Part model, mm, in its own coordinate system. Coordinates: 2 decimals unless noted, no trailing zeros. Loops run counter-clockwise (first coordinate to the right, second up) from the corner with the lowest first, then second, coordinate; pieces in that order, holes last. Notation, with made-up numbers: M 60.5,52.5 L 103.5,52.5 A32 cw 103.5,83.5 Z; hole C -10,11.25 d3. An arc over 180 degrees is marked long. Use a Markdown table: item, result. Add a question column.
1) Pull direction X, two halves, no side cores. Call faces 1 (the flat face through (-1, -15, -47)), 2 (the cylindrical face through (83.624, -14.79, -40.996)): released by +X, released by -X, zero draft, split by the parting line, or undercut.
2) Band-saw the part on C-C (z = 37). State how many separate pieces and enclosed holes the cut face has, plus the area to 3 significant figures.
3) Wall check: probe 1 along X at (y, z) = (-22, 37); probe 2 along Z at (x, y) = (83.8, -11.75); probe 3 along Z at (x, y) = (83, -22). Give the ranges that are in metal, low to high. Write a range as from..to.
4) Band-saw the part on B-B (x = -26). List the corners of the cut face in (y, z), plus the area to 3 significant figures.
5) Band-saw the part on A-A (x = -83.8). List the corners of the cut face in (y, z) (3 decimals).
6) Pin check, flat tip, straight feed: pin 1 Ø8 at (x, z) = (0, 37) entering from +Y (3 decimals). Stop position of the tip, or through.
from build123d import *

# Parameters (mm, degrees)
SKETCH1_W                      = 221.6
SKETCH1_H                      = 94
BOSS_EXTRUDE1_DEPTH            = 30
SKETCH2_R                      = 5.12
CUT_EXTRUDE1_DEPTH             = 125.038864877
CHAMFER1_SIZE                  = 1
M5_TAPPED_HOLE1_D              = 4.2
M5_TAPPED_HOLE1_DEPTH          = 14
M5_TAPPED_HOLE1_TIP            = 1.2618073
M8_TAPPED_HOLE1_AT_2_COUNT     = 2
M8_TAPPED_HOLE1_AT_2_PITCH     = 74
M8_TAPPED_HOLE1_AT_3_COUNT     = 2
M8_TAPPED_HOLE1_AT_3_PITCH     = 214.752322455
M8_TAPPED_HOLE1_AT_4_COUNT     = 2
M8_TAPPED_HOLE1_AT_4_PITCH     = 201.6
M8_TAPPED_HOLE1_AT_5_COUNT     = 2
M8_TAPPED_HOLE1_AT_5_PITCH     = 100.8
M8_TAPPED_HOLE1_AT_6_COUNT     = 2
M8_TAPPED_HOLE1_AT_6_PITCH     = 125.046551332
F_8_0MM_DOWEL_HOLE1_AT_2_COUNT = 2
F_8_0MM_DOWEL_HOLE1_AT_2_PITCH = 183.209606735


with BuildPart() as part:
    # Sketch1 → Boss-Extrude1 (new body)
    with BuildSketch(Plane(origin=(0, 0, 0), x_dir=(1, 0, 0), z_dir=(0, 1, 0))):
        Rectangle(SKETCH1_W, SKETCH1_H)
    extrude(amount=-BOSS_EXTRUDE1_DEPTH)

    # Sketch2 → Cut-Extrude1 (cut, through all)
    with BuildSketch(Plane(origin=(0, 0, 0), x_dir=(1, 0, 0), z_dir=(0, 1, 0))):
        with Locations(Location((35.8, 0, 0), (0, 0, 270))):
            Circle(SKETCH2_R)
        with Locations(Location((73.8, 0, 0), (0, 0, 270))):
            Circle(SKETCH2_R)
        with BuildLine():
            Line((-33.8, 15), (4.2, 15))
            ThreePointArc((4.2, 15), (19.2, 0), (4.2, -15))
            Line((4.2, -15), (-33.8, -15))
            ThreePointArc((-33.8, -15), (-48.8, 0), (-33.8, 15))
        make_face()
    extrude(amount=-CUT_EXTRUDE1_DEPTH, mode=Mode.SUBTRACT)

    # Cut-Sweep1: sweep along a curve in space
    with BuildLine() as cut_sweep1_path:
        ThreePointArc((-33.8, 0, 15), (-48.8, 0, 0), (-33.8, 0, -15))
        Line((-33.8, 0, -15), (4.2, 0, -15))
        ThreePointArc((4.2, 0, -15), (19.2, 0, 0), (4.2, 0, 15))
        Line((4.2, 0, 15), (-33.8, 0, 15))
    # Sketch3 → Cut-Sweep1 (sweep, cut)
    with BuildSketch(Plane(origin=(-14.8, 0, 0), x_dir=(0, 0, -1), z_dir=(1, 0, 0))):
        Polygon((15, -3), (15.707019882, -30), (15, -30), align=None)
    sweep(path=cut_sweep1_path.line, mode=Mode.SUBTRACT)

    # Cut-Sweep2: sweep along a curve in space
    with BuildLine() as cut_sweep2_path:
        ThreePointArc((35.8, 0, 5.12), (39.42038672, 0, 3.62038672), (40.92, 0, 0))
        ThreePointArc((40.92, 0, 0), (39.42038672, 0, -3.62038672), (35.8, 0, -5.12))
        ThreePointArc((35.8, 0, -5.12), (32.17961328, 0, -3.62038672), (30.68, 0, 0))
        ThreePointArc((30.68, 0, 0), (32.17961328, 0, 3.62038672), (35.8, 0, 5.12))
    # Sketch5 → Cut-Sweep2 (sweep, cut)
    with BuildSketch(Plane.XY):
        Polygon((40.92, -3), (41.627019882, -30), (40.92, -30), align=None)
    sweep(path=cut_sweep2_path.line, mode=Mode.SUBTRACT)

    # Cut-Sweep3: sweep along a curve in space
    with BuildLine() as cut_sweep3_path:
        ThreePointArc((73.8, 0, 5.12), (77.42038672, 0, 3.62038672), (78.92, 0, 0))
        ThreePointArc((78.92, 0, 0), (77.42038672, 0, -3.62038672), (73.8, 0, -5.12))
        ThreePointArc((73.8, 0, -5.12), (70.17961328, 0, -3.62038672), (68.68, 0, 0))
        ThreePointArc((68.68, 0, 0), (70.17961328, 0, 3.62038672), (73.8, 0, 5.12))
    # Sketch9 → Cut-Sweep3 (sweep, cut)
    with BuildSketch(Plane.XY):
        Polygon((78.92, -3), (79.627019882, -30), (78.92, -30), align=None)
    sweep(path=cut_sweep3_path.line, mode=Mode.SUBTRACT)

    # Chamfer1
    chamfer1_edges = [part.edges().sort_by_distance(p)[0] for p in [
        (-110.8, -30, 0),
        (0, -30, 47),
        (110.8, -30, 0),
        (0, 0, 47),
        (-110.8, 0, 0),
        (0, 0, -47),
        (110.8, 0, 0),
        (110.8, -15, 47),
        (-110.8, -15, 47),
        (-110.8, -15, -47),
        (0, -30, -47),
    ]]
    chamfer(chamfer1_edges, length=CHAMFER1_SIZE)

    # M5 Tapped Hole1
    with Locations(Plane.XY.offset(47)):
        with Locations((14.45, -7)):
            Hole(M5_TAPPED_HOLE1_D / 2, depth=M5_TAPPED_HOLE1_DEPTH)
            with Locations((0, 0, -(M5_TAPPED_HOLE1_DEPTH + M5_TAPPED_HOLE1_TIP / 2))):  # 118° drill point
                Cone(0, M5_TAPPED_HOLE1_D / 2, M5_TAPPED_HOLE1_TIP, mode=Mode.SUBTRACT)

    # Sketch15 → M8 Tapped Hole1 (revolve, cut)
    with BuildSketch(Plane(origin=(-100.8, 0, 37), x_dir=(0, 0, 1), z_dir=(1, 0, 0))):
        Polygon((0, 0), (0, 30), (4.025, 30), (3.4, 29.375), (3.4, 0.625), (4.025, 0), align=None)
    m8_tapped_hole1 = revolve(axis=Axis((-100.8, 6.35, 37), (0, -1, 0)), mode=Mode.SUBTRACT)

    # M8 Tapped Hole1 at 2: M8 Tapped Hole1 ×2
    with Locations(*[(0, 0, -i * M8_TAPPED_HOLE1_AT_2_PITCH) for i in range(1, M8_TAPPED_HOLE1_AT_2_COUNT)]):
        add(m8_tapped_hole1, mode=Mode.SUBTRACT)

    # M8 Tapped Hole1 at 3: M8 Tapped Hole1 ×2
    with Locations(*[Vector(0.9387558546280332, 0, -0.34458300219481375) * (i * M8_TAPPED_HOLE1_AT_3_PITCH) for i in range(1, M8_TAPPED_HOLE1_AT_3_COUNT)]):
        add(m8_tapped_hole1, mode=Mode.SUBTRACT)

    # M8 Tapped Hole1 at 4: M8 Tapped Hole1 ×2
    with Locations(*[(i * M8_TAPPED_HOLE1_AT_4_PITCH, 0, 0) for i in range(1, M8_TAPPED_HOLE1_AT_4_COUNT)]):
        add(m8_tapped_hole1, mode=Mode.SUBTRACT)

    # M8 Tapped Hole1 at 5: M8 Tapped Hole1 ×2
    with Locations(*[(i * M8_TAPPED_HOLE1_AT_5_PITCH, 0, 0) for i in range(1, M8_TAPPED_HOLE1_AT_5_COUNT)]):
        add(m8_tapped_hole1, mode=Mode.SUBTRACT)

    # M8 Tapped Hole1 at 6: M8 Tapped Hole1 ×2
    with Locations(*[Vector(0.8060997998454218, 0, -0.591779614965885) * (i * M8_TAPPED_HOLE1_AT_6_PITCH) for i in range(1, M8_TAPPED_HOLE1_AT_6_COUNT)]):
        add(m8_tapped_hole1, mode=Mode.SUBTRACT)

    # Sketch17 → Ø8.0mm Dowel Hole1 (revolve, cut)
    with BuildSketch(Plane(origin=(-83.8, 0, 37), x_dir=(0, 0, 1), z_dir=(1, 0, 0))):
        Polygon((0, 0), (0, 30), (4.025, 30), (4, 29.975), (4, 0.025), (4.025, 0), align=None)
    f_8_0mm_dowel_hole1 = revolve(axis=Axis((-83.8, 6.35, 37), (0, -1, 0)), mode=Mode.SUBTRACT)

    # Ø8.0mm Dowel Hole1 at 2: Ø8.0mm Dowel Hole1 ×2
    with Locations(*[Vector(0.9147991908656035, 0, -0.40390895062085114) * (i * F_8_0MM_DOWEL_HOLE1_AT_2_PITCH) for i in range(1, F_8_0MM_DOWEL_HOLE1_AT_2_COUNT)]):
        add(f_8_0mm_dowel_hole1, mode=Mode.SUBTRACT)

    # Mirror1: Ø8.0mm Dowel Hole1 across plane
    add(f_8_0mm_dowel_hole1.mirror(Plane.XY), mode=Mode.SUBTRACT)

    # Mirror1 copy 1 sketch → Mirror1 copy 1 (revolve, cut)
    with BuildSketch(Plane(origin=(83.8, 0, 37), x_dir=(0, 0, -1), z_dir=(1, 0, 0))):
        Polygon((0, 0), (0, -30), (4.025, -30), (4, -29.975), (4, -0.025), (4.025, 0), align=None)
    revolve(axis=Axis((83.8, 6.35, 37), (0, 1, 0)), mode=Mode.SUBTRACT)


solid = part.part
Entries:
| question | item | result |
|---|---|---|
| 1 | face 1 | zero draft |
| 1 | face 2 | undercut |
| 2 | separate pieces | 6 |
| 2 | enclosed holes | 1 |
| 2 | area | 5,540 mm2 |
| 3 | probe 1 | -110.8..-104.2, -97.4..-87.8, -79.8..-3.4, 3.4..79.8, 87.8..97.4, 104.2..110.8 |
| 3 | probe 2 | -47..-41, -33..33, 41..47 |
| 3 | probe 3 | -47..-40.92, -33.08..33.08, 40.92..47 |
| 4 | outline | M -30,-46 L -29,-47 L -1,-47 L 0,-46 L 0,-15 L -3,-15 L -30,-15.71 Z; M -30,15.71 L -3,15 L 0,15 L 0,46 L -1,47 L -29,47 L -30,46 Z |
| 4 | area | 1,900 mm2 |
| 5 | outline | M -30,-46 L -29,-47 L -1,-47 L 0,-46 L 0,-41.025 L -0.025,-41 L -29.975,-41 L -30,-41.025 Z; M -30,-32.975 L -29.975,-33 L -0.025,-33 L 0,-32.975 L 0,32.975 L -0.025,33 L -29.975,33 L -30,32.975 Z; M -30,41.025 L -29.975,41 L -0.025,41 L 0,41.025 L 0,46 L -1,47 L -29,47 L -30,46 Z |
| 6 | pin 1 | y = -0.025 |
